Geometry: final body of the model. Coordinates: model frame, mm. A direction names the side the tool comes from. Coordinates: 2 decimals unless noted, no trailing zeros. Order: outer loops, then holes, each group sorted by start corner. A loop starts at its lowest first (then second) coordinate and runs counter-clockwise, first axis right, second up. Notation, with made-up numbers: M 19,-27.75 L 35,-27.75 A16 ccw 35,-5.75 Z; hole C 85.25,4.5 d6. An arc over 180 degrees is marked long. Write item = value, one per line.
Autodesk Inventor part; units mm, degrees
ref_plane "YZ Plane" through (0, 0, 0) normal (1, 0, 0) x (0, 1, 0)
ref_plane "XZ Plane" through (0, 0, 0) normal (0, 1, 0) x (-1, 0, 0)
ref_plane "XY Plane" through (0, 0, 0) normal (0, 0, 1) x (1, 0, 0)
sketch "Sketch1" plane through (0, 0, 0) normal (0, 0, 1) x (1, 0, 0)
  line L0 (0, 0) -> (0, 3)
  line L1 (0, 3) -> (1, 3)
  line L2 (1, 3) -> (1, 1.75)
  line L3 (0, 0) -> (14, 0)
  line L4 (1, 1.75) -> (9.5, 1.75)
  line L5 (9.5, 1.75) -> (9.5, 1.6)
  line L6 (9.5, 1.6) -> (11, 1.6)
  line L7 (11, 1.6) -> (11, 1.3)
  line L8 (11, 1.3) -> (14, 1.5)
  line L9 (14, 1.5) -> (15.2, 0.6)
  line L10 (15.2, 0.6) -> (15.2, 0)
  line L11 (0, 1.5) -> (-8.6528, 1.5)
  line L12 (-8.6528, 1.5) -> (-8.6528, 0)
  line L13 (0, 0) -> (-8.6528, 0)
  line L14 (14, 0) -> (15.2, 0)
  dimension "d1" = 1
  dimension "d3" = 14
  dimension "d5" = 6
  dimension "d6" = 3.5
  dimension "d7" = 3.2
  dimension "d8" = 2.6
  dimension "d9" = 3
  dimension "d11" = 14
  dimension "d12" = 11
  dimension "d13" = 9.5
  dimension "d15" = 1.2
  dimension "d16" = 1.2
  dimension "d17" = 8.6528
revolve "Revolution1" add sketch "Sketch1" angle 360 about axis through (0, 0, 0) along (1, 0, 0)
properties part number "3,5mm jack"
1) Section D-D, the plane x = 9.75. Return loops of the section in (y, z), and give its area (3 significant figures).
Numbers:
outline = C 0,0 d3.2
area = 8.04 mm²
2) Section A-A, the plane y = 0. Return loops of the section in (x, z), and give its area (3 significant figures).
Numbers:
outline = M -8.65,-1.5 L 0,-1.5 L 0,-3 L 1,-3 L 1,-1.75 L 9.5,-1.75 L 9.5,-1.6 L 11,-1.6 L 11,-1.3 L 14,-1.5 L 15.2,-0.6 L 15.2,0.6 L 14,1.5 L 11,1.3 L 11,1.6 L 9.5,1.6 L 9.5,1.75 L 1,1.75 L 1,3 L 0,3 L 0,1.5 L -8.65,1.5 Z
area = 77.4 mm²
3) Line query: L1, parallel to X at y = -0.2, z = -1.65; L2, parallel to X at y = -2.4, z = -1.4; L3, parallel to Y at x = 8.25, z = 0.05. Output: solid intervals per line, ascending.
Numbers:
L1 = 0 to 9.5
L2 = 0 to 1
L3 = -1.75 to 1.75
4) Pin query (flat end, axial travel): pin 1 (2 mm diameter, centred on y = 2, z = 2, fed in from +X); pin 2 (1 mm diameter, centred on x = 5.5, z = -0.5, fed in from +Y); pin 3 (2 mm diameter, centred on x = 5, z = 2, fed in from -Y). Return the tip coordinate at first contact, or that it passes through.
Numbers:
pin_1 = 1
pin_2 = 1.75
pin_3 = -1.44
5) Set-up query: faces 1 (the face through (0, 1.3, -1.3)), 2 (the face through (1, 0, -2)), 3 (the face through (12.521, 1.337, 0.421)), 4 (the face through (-8.653, 0, 0)). Return all of +Z, -Z, +X, -X, +Y, -Y with unobstructed straight access to the full face (end or side cutting, diameter ignored); none if empty.
Numbers:
face_1 = -X
face_2 = +X
face_3 = none
face_4 = +Z, -Z, -X, +Y, -Y
6) Section C-C, the plane x = 6.25. Return loops of the section in (y, z), and give its area (3 significant figures).
Numbers:
outline = C 0,0 d3.5
area = 9.62 mm²
